The model under review builds one solid part; all positions refer to its coordinate system, in mm. Face numbers are marked on the shaded views. A direction names the side the tool comes from. Give positions to 0.01 mm unless a question says otherwise; leave off trailing zeros. Loops run counter-clockwise (first coordinate to the right, second up) from the corner with the lowest first, then second, coordinate; pieces in that order, holes last. Notation, with made-up numbers: (64.5, -2.75) - (70.5, -2.75) arc R30 ccw to (70.5, 30.25) - close; hole circle Ø9 at (24.5, 21.25). An arc over 180 degrees is marked (long way). Answer as a JSON object with one key per item and string values.
from build123d import *

# Parameters (mm, degrees)
SKETCH1_R           = 1.1
BOSS_EXTRUDE1_DEPTH = 1.5
SKETCH2_R           = 2.5
BOSS_EXTRUDE2_DEPTH = 1
BOSS_EXTRUDE3_DEPTH = 4
SKETCH4_W           = 6
SKETCH4_H           = 14
SKETCH4_R           = 1.1
BOSS_EXTRUDE4_DEPTH = 5
FILLET4_R           = 3
FILLET1_R           = 0.5
SKETCH5_R           = 1.75
CUT_EXTRUDE1_DEPTH  = 4
FILLET3_R           = 2


with BuildPart() as part:
    # Sketch1 → Boss-Extrude1 (new body)
    with BuildSketch(Plane.XY):
        with BuildLine():
            Line((-15, 7), (0, 7))
            ThreePointArc((0, 7), (7, 0), (0, -7))
            Line((0, -7), (-15, -7))
            Line((-15, -7), (-15, 7))
        make_face()
        with Locations((-12, 3.5)):
            Circle(SKETCH1_R, mode=Mode.SUBTRACT)
        with Locations((-12, -3.5)):
            Circle(SKETCH1_R, mode=Mode.SUBTRACT)
    extrude(amount=BOSS_EXTRUDE1_DEPTH)

    # Sketch2 → Boss-Extrude2 (add)
    with BuildSketch(Plane(origin=(0, 0, 0), x_dir=(-1, 0, 0), z_dir=(0, 0, -1))):
        Circle(SKETCH2_R)
    extrude(amount=BOSS_EXTRUDE2_DEPTH)

    # Sketch3 → Boss-Extrude3 (add)
    with BuildSketch(Plane(origin=(0, 0, -1), x_dir=(-1, 0, 0), z_dir=(0, 0, -1))):
        with BuildLine():
            Line((1.13862177, 1.394109201), (1.13862177, -1.394109201))
            ThreePointArc((1.13862177, -1.394109201), (-1.8, 0), (1.13862177, 1.394109201))
        make_face()
    extrude(amount=BOSS_EXTRUDE3_DEPTH)

    # Sketch4 → Boss-Extrude4 (add)
    with BuildSketch(Plane(origin=(0, 0, 0), x_dir=(-1, 0, 0), z_dir=(0, 0, -1))):
        with Locations((12, 0)):
            Rectangle(SKETCH4_W, SKETCH4_H)
        with Locations((12, 3.5)):
            Circle(SKETCH4_R, mode=Mode.SUBTRACT)
        with Locations((12, -3.5)):
            Circle(SKETCH4_R, mode=Mode.SUBTRACT)
    extrude(amount=BOSS_EXTRUDE4_DEPTH)

    # Fillet4
    fillet4_edges = [part.edges().sort_by_distance(p)[0] for p in [
        (-15, -7, -1.75),
        (-15, 7, -1.75),
    ]]
    fillet(fillet4_edges, radius=FILLET4_R)

    # Fillet1
    fillet1_edges = [part.edges().sort_by_distance(p)[0] for p in [
        (7, 0, 1.5),
        (-15, 0, 1.5),
        (-6, -7, 1.5),
        (-14.121320344, -6.121320344, 1.5),
        (-14.121320344, 6.121320344, 1.5),
        (-6, 7, 1.5),
    ]]
    fillet(fillet1_edges, radius=FILLET1_R)

    # Sketch5 → Cut-Extrude1 (cut)
    with BuildSketch(Plane.XY.offset(1.5)):
        with Locations((-12, 3.5)):
            Circle(SKETCH5_R)
        with Locations((-12, -3.5)):
            Circle(SKETCH5_R)
    extrude(amount=-CUT_EXTRUDE1_DEPTH, mode=Mode.SUBTRACT)

    # Fillet3
    fillet3_edges = [part.edges().sort_by_distance(p)[0] for p in [
        (-9, 0, 0),
    ]]
    fillet(fillet3_edges, radius=FILLET3_R)


solid = part.part
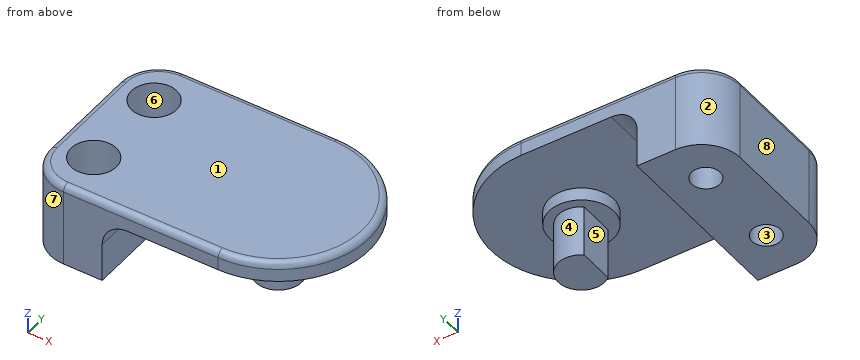
Q1. For the marked faces 4, 5, 6, 7 and 8, list the 3-axis set-ups (+Z, -Z, +X, -X, +Y, -Y) from which the entire face can be reached by the end or side of a thin tool; tool diameter is ignored.
Results:
{"face 4": "-Z", "face 5": "-Z, +Y, -Y", "face 6": "+Z", "face 7": "+Z, -Z, -X, -Y", "face 8": "+Z, -Z, -X, +Y, -Y"}
Q2. The part is to be moulded in two halves that separate along X. For the marked faces 1, 2 and 3, say which applies: +X half, -X half, draft (parallel to the pull), parting line (faces both ways), or undercut.
Results:
{"face 1": "draft", "face 2": "-X half", "face 3": "undercut"}
Q3. To check wall thickness, follow probe 1 along Y at (x, z) = (-12, -3.15); probe 2 along Y at (x, z) = (-12, 0.4); probe 3 along X at (y, z) = (-3.5, -3.1). State the ranges of each line that lie inside material, in increasing order. Write a range as [from, to].
Results:
{"probe 1": "y = [-7, -4.6], [-2.4, 2.4], [4.6, 7]", "probe 2": "y = [-7, -5.25], [-1.75, 1.75], [5.25, 7]", "probe 3": "x = [-15, -13.1], [-10.9, -9]"}
Q4. Consider section C-C, the plane x = -5. State the section outline as (y, z) points.
Results:
{"outline": "(-7, 0) - (7, 0) - (7, 1) arc R0.5 ccw to (6.5, 1.5) - (-6.5, 1.5) arc R0.5 ccw to (-7, 1) - close"}
Q5. Consider section D-D, the plane x = -0.25. State the section outline as (y, z) points, plus the area to 3 significant figures.
Results:
{"outline": "(-7, 0) - (-2.49, 0) - (-2.49, -1) - (-1.78, -1) - (-1.78, -5) - (1.78, -5) - (1.78, -1) - (2.49, -1) - (2.49, 0) - (7, 0) - (7, 1) arc R0.5 ccw to (6.5, 1.5) - (-6.5, 1.5) arc R0.5 ccw to (-7, 1) - close", "area": "40.1 mm^2"}
Q6. Clearance check with flat-ended pins moving along their axes: pin 1 Ø1.8 at (x, y) = (-12, 3.5) entering from +Z; pin 2 Ø2.5 at (y, z) = (-2, -3) entering from +X. State where each tip first meets the part, or that it passes through.
Results:
{"pin 1": "passes through", "pin 2": "stops at x = 1.64"}
Q7. Consider section A-A, the plane z = -2.75. State the section outline as (x, y) points.
Results:
{"outline": "(-15, -4) arc R3 ccw to (-12, -7) - (-9, -7) - (-9, 7) - (-12, 7) arc R3 ccw to (-15, 4) - close; (-1.14, -1.39) arc R1.8 ccw (long way) to (-1.14, 1.39) - close; hole circle Ø2.2 at (-12, -3.5); hole circle Ø2.2 at (-12, 3.5)"}
Q8. Consider section B-B, the plane y = 0. State the section outline as (x, z) points, plus the area to 3 significant figures.
Results:
{"outline": "(-15, -5) - (-9, -5) - (-9, -2) arc R2 cw to (-7, 0) - (-2.5, 0) - (-2.5, -1) - (-1.14, -1) - (-1.14, -5) - (1.8, -5) - (1.8, -1) - (2.5, -1) - (2.5, 0) - (7, 0) - (7, 1) arc R0.5 ccw to (6.5, 1.5) - (-14.5, 1.5) arc R0.5 ccw to (-15, 1) - close", "area": "80.5 mm^2"}
